Could you check a few things on this model? Use its own coordinates, in mm. A direction names the side the tool comes from. Give positions to 0.01 mm unless a question says otherwise; leave off trailing zeros. Loops run counter-clockwise (first coordinate to the right, second up) from the corner with the lowest first, then second, coordinate; pieces in that order, holes last. Notation, with made-up numbers: M 13.5,85.25 L 68.5,85.25 A7 cw 68.5,89.25 Z; hole C 12.25,33 d5. An arc over 180 degrees is marked long. Use CSV: the item, a comma, the result in double quotes.
```python
from build123d import *

# Parameters (mm, degrees)
SKETCH1_R             = 9.4615
EXTRUDE1_DEPTH        = 3.175
SKETCH2_R             = 7.8232
EXTRUDE2_DEPTH        = 9.525
F_6_32_TAPPED_HOLE2_D = 2.7051


with BuildPart() as part:
    # Sketch1 → Extrude1 (new body)
    with BuildSketch(Plane(origin=(0, 0, 0), x_dir=(1, 0, 0), z_dir=(0, 1, 0))):
        with Locations(Location((0, 0, 0), (0, 0, 270))):  # turned: the seam where the file's is
            Circle(SKETCH1_R)
    extrude(amount=EXTRUDE1_DEPTH)

    # Sketch2 → Extrude2 (add)
    with BuildSketch(Plane(origin=(0, 3.175, 0), x_dir=(1, 0, 0), z_dir=(0, 1, 0))):
        with Locations(Location((0, 0, 0), (0, 0, 270))):  # turned: the seam where the file's is
            Circle(SKETCH2_R)
    extrude(amount=EXTRUDE2_DEPTH)

    # #6-32 Tapped Hole2 (through all)
    with Locations(Plane(origin=(0, 0, 0), x_dir=(0, 0, -1), z_dir=(0, -1, 0))):
        with Locations((0, 0)):
            Hole(F_6_32_TAPPED_HOLE2_D / 2)


solid = part.part
```
1. I want a section at D-D, the plane z = -4.5. List the corners of the cut face in (x, y) for me (3 decimals), then the cut area to 3 significant figures.
Outcome:
outline,"M -8.323,0 L 8.323,0 L 8.323,3.175 L 6.399,3.175 L 6.399,12.7 L -6.399,12.7 L -6.399,3.175 L -8.323,3.175 Z"
area,"175 mm2"
2. I want a section at B-B, the plane x = 0. List the corners of the cut face in (y, z) for me (1 decimal), then the cut area to 3 significant figures.
Outcome:
outline,"M 0,-9.5 L 3.2,-9.5 L 3.2,-7.8 L 12.7,-7.8 L 12.7,-1.4 L 0,-1.4 Z; M 0,1.4 L 12.7,1.4 L 12.7,7.8 L 3.2,7.8 L 3.2,9.5 L 0,9.5 Z"
area,"175 mm2"
3. I want a section at A-A, the plane z = 0. List the corners of the cut face in (x, y) for me (1 decimal), then the cut area to 3 significant figures.
Outcome:
outline,"M -9.5,0 L -1.4,0 L -1.4,12.7 L -7.8,12.7 L -7.8,3.2 L -9.5,3.2 Z; M 1.4,0 L 9.5,0 L 9.5,3.2 L 7.8,3.2 L 7.8,12.7 L 1.4,12.7 Z"
area,"175 mm2"
4. If we mould it in two halves opening along Z, with no side actions, what happens to faces 1 (the face through (0, 12.7, 2)), 2 (the face through (0.41, 6.44, 1.29)), 3 (the face through (2.35, 7.87, 7.46))? For each: +Z half, -Z half, draft (parallel to the pull), parting line (faces both ways), or undercut.
Outcome:
face 1,"draft"
face 2,"undercut"
face 3,"parting line"
5. I'm going to push flat-ended pins straight in: pin 1 Ø1 at (x, y) = (-1.5, 3.5) entering from -Z (3 decimals); pin 2 Ø1 at (y, z) = (4, -6.5) entering from -X; pin 3 Ø1.5 at (y, z) = (10, 1.5) entering from -X. Where does each tip first touch, or does it pass through?
Outcome:
pin 1,"z = -9.395"
pin 2,"x = -5.02"
pin 3,"x = -7.79"
6. I want a section at C-C, the plane y = 7.75. List the corners of the cut face in (x, z) for me, then the cut area to 3 significant figures.
Outcome:
outline,"C 0,0 d15.65; hole C 0,0 d2.71"
area,"187 mm2"
7. Which directions (+Z, -Z, +X, -X, +Y, -Y) give clear straight access to the entire face, cutting with the end or side of a thin tool? Please do faces 4 (the face through (7, 3.175, -4)), 5 (the face through (2.842, 1.565, 9.025)).
Outcome:
face 4,"+Y"
face 5,"+Y, -Y"
8. Please list where these lines run through material, in increasing order: line 1 (X direction, y = 8.5, z = 0); line 2 (Y direction, x = -2.75, z = -8.25) (3 decimals); line 3 (Z direction, x = 3, y = 8.75).
Outcome:
line 1,"-7.82 to -1.35, 1.35 to 7.82"
line 2,"0 to 3.175"
line 3,"-7.23 to 7.23"
